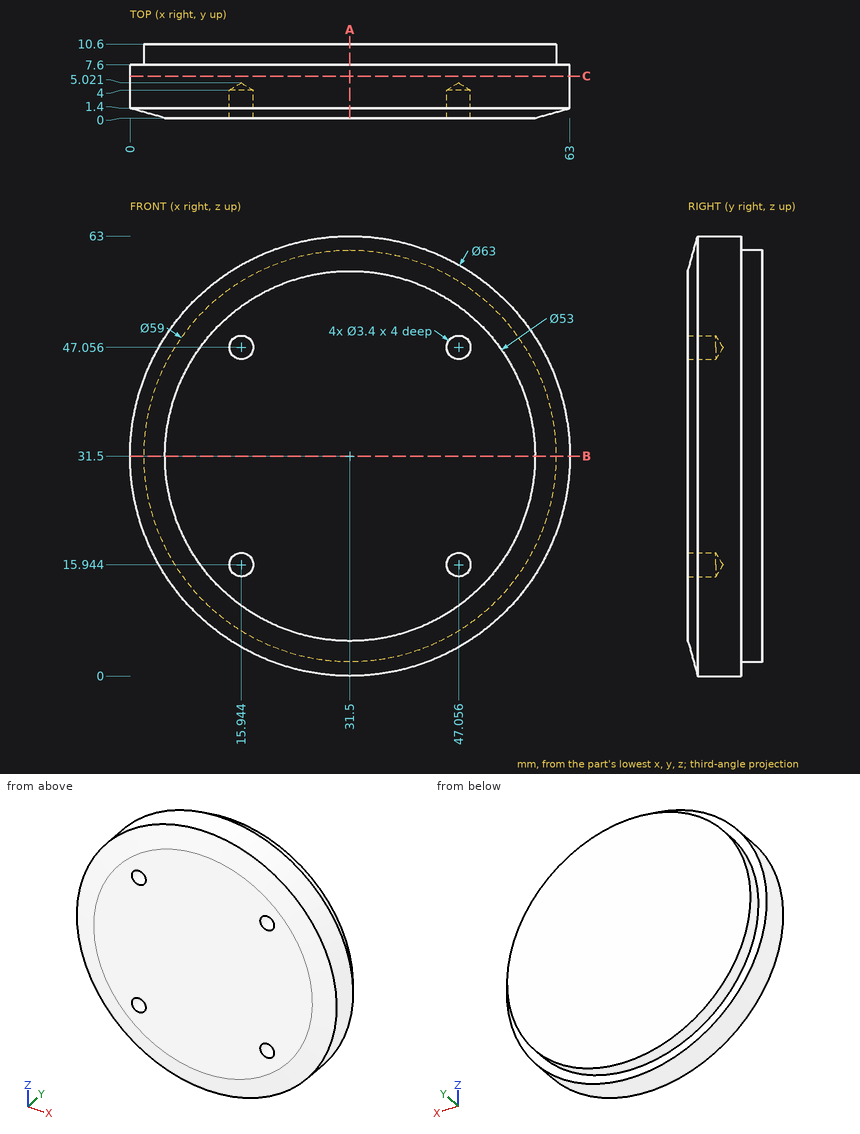
Geometry check sheet. Reference: drawing and pictorial views, mm from the part's lowest x, y, z. Round coordinates to 2 decimals unless told otherwise and drop trailing zeros. Loops run counter-clockwise (first coordinate to the right, second up) from the corner with the lowest first, then second, coordinate; pieces in that order, holes last. Notation, with made-up numbers: (-8.5, 56) - (20.5, 56) arc R14 cw to (20.5, 83) - close; hole circle Ø10 at (22.5, 33). An arc over 180 degrees is marked (long way). Use a Markdown table: item, result. Add a question column.
1. Gauge pin test, flat ends, axial feed: pin 1 (1.5 mm diameter, centred on y = 8.5, z = 22.5, fed in from -X); pin 2 (5 mm diameter, centred on x = 7.5, z = 54, fed in from +Y); pin 3 (6 mm diameter, centred on y = 3, z = 35.5, fed in from +X); pin 4 (1 mm diameter, centred on x = 31, y = 7.5, fed in from +Z). Record the tip position at first contact, or that the pin passes through.
2. Section check A-A, the plane x = 31.5. Record the boundary of the cut face in (y, z), plus the area to 3 significant figures.
3. Thickness scan on probe 1 along X at (y, z) = (7.75, 29); probe 2 along Z at (x, y) = (44, 4.5) (1 decimal); probe 3 along X at (y, z) = (1.75, 34). Record the ranges inside material, lowest first. Write a range as [from, to].
4. Section check C-C, the plane y = 6. Record the boundary of the cut face in (x, z).
5. Section check B-B, the plane z = 31.5. Record the boundary of the cut face in (x, y), plus the area to 3 significant figures.
Checks:
| question | item | result |
|---|---|---|
| 1 | pin 1 | stops at x = 3.18 |
| 1 | pin 2 | stops at y = 7.6 |
| 1 | pin 3 | stops at x = 62.98 |
| 1 | pin 4 | stops at z = 63 |
| 2 | outline | (0, 5) - (1.4, 0) - (7.6, 0) - (7.6, 2) - (10.6, 2) - (10.6, 61) - (7.6, 61) - (7.6, 63) - (1.4, 63) - (0, 58) - close |
| 2 | area | 649 mm^2 |
| 3 | probe 1 | x = [2.11, 60.89] |
| 3 | probe 2 | z = [2.6, 60.4] |
| 3 | probe 3 | x = [0.1, 62.9] |
| 4 | outline | circle Ø63 at (31.5, 31.5) |
| 5 | outline | (0, 1.4) - (5, 0) - (58, 0) - (63, 1.4) - (63, 7.6) - (61, 7.6) - (61, 10.6) - (2, 10.6) - (2, 7.6) - (0, 7.6) - close |
| 5 | area | 649 mm^2 |
